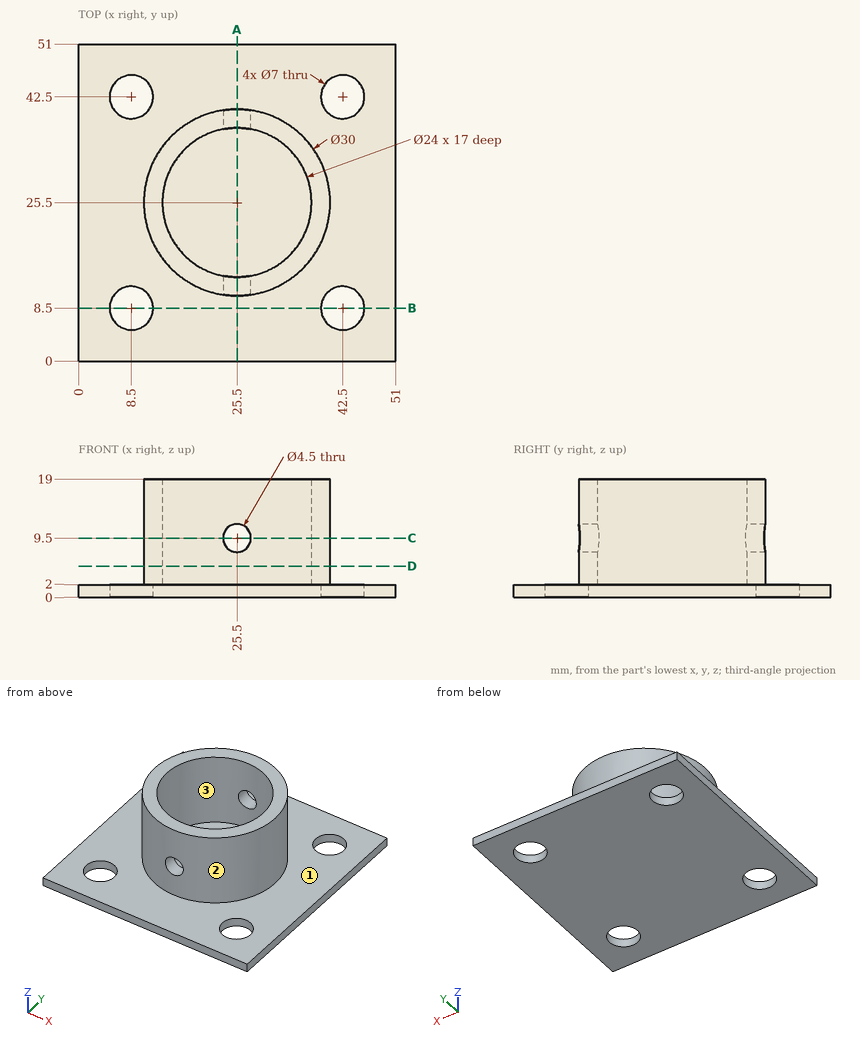
Check sheet for the drawn part. Datum: minimum x, y, z corner. Units: mm. Coordinates: 2 decimals unless noted, no trailing zeros. Order: outer loops, then holes, each group sorted by start corner. A loop starts at its lowest first (then second) coordinate and runs counter-clockwise, first axis right, second up. Notation, with made-up numbers: (-11.5, 21.5) -> (46.5, 21.5) arc R30 cw to (46.5, 44.5) -> close; hole circle Ø11 at (-29, -2.5). An arc over 180 degrees is marked (long way). Use a Markdown table: item, result. Add a question column.
1. Cross-section at C-C (z = 9.5). Enter the section's corners in (x, y), and give its area (3 significant figures).
2. Cross-section at A-A (x = 25.5). Enter the section's corners in (y, z), and give its area (3 significant figures).
3. Mould release check, pull along X, two halves, no side actions. Record for the marked faces 1, 2 and 3: pulls with the +X half, pulls with the -X half, needs draft (parallel to the pull), parting line crosses it, or undercut.
4. Material ranges on L1, parallel to Y at x = 8.5, z = 1; L2, parallel to Y at x = 25.5, z = 7; L3, parallel to Z at x = 27, y = 34, recorded low to high.
5. Go/stop test with flat-tipped pins: pin 1 Ø1 at (y, z) = (23, 4) entering from -X; pin 2 Ø7 at (x, y) = (30, 24) entering from +Z; pin 3 Ø4 at (x, z) = (25.5, 9.5) entering from -Y; pin 4 Ø1 at (y, z) = (11.5, 7.5) entering from +X. Record where each tip stops, or that it passes through.
6. Cross-section at B-B (y = 8.5). Enter the section's corners in (x, z), and give its area (3 significant figures).
7. Cross-section at D-D (z = 5). Enter the section's corners in (x, y), and give its area (3 significant figures).
Filled sheet:
| question | item | result |
|---|---|---|
| 1 | outline | (23.25, 10.67) -> (23.25, 13.71) arc R12 cw to (23.25, 37.29) -> (23.25, 40.33) arc R15 ccw to start; (27.75, 10.67) arc R15 ccw to (27.75, 40.33) -> (27.75, 37.29) arc R12 cw to (27.75, 13.71) -> close |
| 1 | area | 227 mm2 |
| 2 | outline | (0, 0) -> (51, 0) -> (51, 2) -> (40.5, 2) -> (40.5, 7.25) -> (37.5, 7.25) -> (37.5, 2) -> (13.5, 2) -> (13.5, 7.25) -> (10.5, 7.25) -> (10.5, 2) -> (0, 2) -> close; (10.5, 11.75) -> (13.5, 11.75) -> (13.5, 19) -> (10.5, 19) -> close; (37.5, 11.75) -> (40.5, 11.75) -> (40.5, 19) -> (37.5, 19) -> close |
| 2 | area | 177 mm2 |
| 3 | face 1 | needs draft |
| 3 | face 2 | parting line crosses it |
| 3 | face 3 | undercut |
| 4 | L1 | 0 to 5, 12 to 39, 46 to 51 |
| 4 | L2 | 10.5 to 13.5, 37.5 to 40.5 |
| 4 | L3 | 0 to 2 |
| 5 | pin 1 | x = 10.63 |
| 5 | pin 2 | z = 2 |
| 5 | pin 3 | through |
| 5 | pin 4 | x = 32.04 |
| 6 | outline | (0, 0) -> (5, 0) -> (5, 2) -> (0, 2) -> close; (12, 0) -> (39, 0) -> (39, 2) -> (12, 2) -> close; (46, 0) -> (51, 0) -> (51, 2) -> (46, 2) -> close |
| 6 | area | 74.0 mm2 |
| 7 | outline | circle Ø30 at (25.5, 25.5); hole circle Ø24 at (25.5, 25.5) |
| 7 | area | 254 mm2 |
